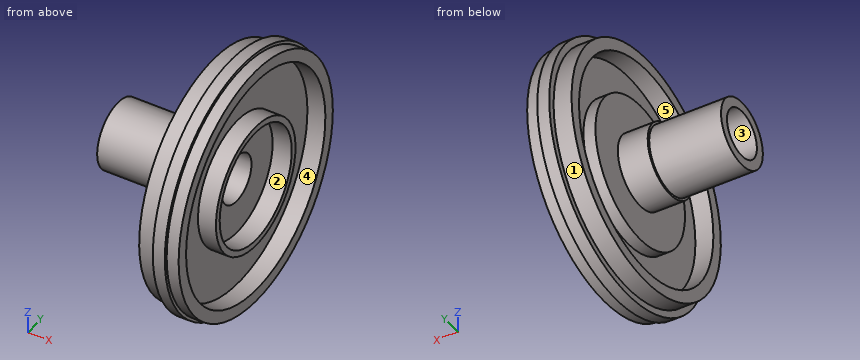
```python
from build123d import *


with BuildPart() as part:
    # Sketch1 → Revolve1 (revolve)
    with BuildSketch(Plane.XY, mode=Mode.PRIVATE) as revolve1_sk:
        Polygon((0, 6.35), (31.4198, 6.35), (31.4198, 15.33525), (36.4998, 15.33525), (36.4998, 16.92275), (31.7373, 16.92275), (31.7373, 29.62275), (36.4998, 29.62275), (36.4998, 32.79775), (33.3248, 32.79775), (33.3248, 33.5915), (30.1498, 33.5915), (30.1498, 31.75), (25.3873, 31.75), (25.3873, 28.575), (30.1498, 28.575), (30.1498, 19.05), (26.9748, 19.05), (26.9748, 9.525), (19.05, 9.525), (19.05, 8.89), (0, 8.89), align=None)
    revolve(revolve1_sk.sketch.rotate(Axis((0, 0, 0), (1, 0, 0)), 90), axis=Axis((0, 0, 0), (1, 0, 0)))


solid = part.part
```
Model file for the job. Use its own axes, mm. Face numbers are marked on the shaded views. A direction names the side the tool comes from. Coordinates: 2 decimals unless noted, no trailing zeros. Order: outer loops, then holes, each group sorted by start corner. A loop starts at its lowest first (then second) coordinate and runs counter-clockwise, first axis right, second up. Notation, with made-up numbers: (8.25, 32.25) - (12.25, 32.25) arc R20 cw to (12.25, 62.25) - close; hole circle Ø5 at (29, 24). An arc over 180 degrees is marked (long way). Return JSON: item names as keys, results as strings. Group by question number.
1) Saw through at D-D, the plane y = 18. Write the cut outline in (x, z).
2) Tool access for the marked faces 3, 4 and 5: list every direction of +Z, -Z, +X, -X, +Y, -Y with a clear straight run to the whole face (end or side of a thin tool).
3) Saw through at B-B, the plane x = 17.5. Write the cut outline in (y, z), plus the area to 3 significant figures.
4) Probe line 1 (Y direction, x = 33.8, z = 0); line 2 (Y direction, x = 33, z = 0); line 3 (Z direction, x = 26, y = -8.5). List the from-to ranges inside material, lowest first. Write a range as from..to.
5) Flat gauge pins, fed straight in: P1, Ø6, axis at y = 20, z = 15.5, coming from the -X side; P2, Ø1, axis at x = 24.5, y = 5.5, coming from the +Z side; P3, Ø6, axis at x = 4.5, y = 8, coming from the -Z side. Where does each tip first touch, or does it go through?
6) Saw through at C-C, the plane z = -26.5. Write the cut outline in (x, y).
7) Saw through at A-A, the plane x = 29. Write the cut outline in (y, z) (3 decimals), plus the area to 3 significant figures.
8) Mould opens along Z. For the marked faces 1 and 2 say: released by +Z, released by -Z, zero draft, split by the parting line, or undercut.
Values found:
{
 "1": {"outline": "(25.39, -26.15) - (30.15, -26.15) - (30.15, -28.36) - (33.32, -28.36) - (33.32, -27.42) - (36.5, -27.42) - (36.5, -23.53) - (31.74, -23.53) - (31.74, 23.53) - (36.5, 23.53) - (36.5, 27.42) - (33.32, 27.42) - (33.32, 28.36) - (30.15, 28.36) - (30.15, 26.15) - (25.39, 26.15) - (25.39, 22.19) - (30.15, 22.19) - (30.15, 6.24) - (26.97, 6.24) - (26.97, -6.24) - (30.15, -6.24) - (30.15, -22.19) - (25.39, -22.19) - close"},
 "2": {"face 3": "+X, -X", "face 4": "+X", "face 5": "-X"},
 "3": {"outline": "circle Ø17.78 at (0, 0); hole circle Ø12.7 at (0, 0)", "area": "122 mm²"},
 "4": {"line 1": "y = -32.8..-29.62, -16.92..-15.34, 15.34..16.92, 29.62..32.8", "line 2": "y = -33.59..-29.62, -16.92..-15.34, 15.34..16.92, 29.62..33.59", "line 3": "z = -30.59..-27.28, -4.3..4.3, 27.28..30.59"},
 "5": {"P1": "stops at x = 30.15", "P2": "stops at z = 8.11", "P3": "stops at z = -7.35"},
 "6": {"outline": "(25.39, -17.49) - (30.15, -17.49) - (30.15, -20.64) - (33.32, -20.64) - (33.32, -19.32) - (36.5, -19.32) - (36.5, -13.24) - (31.74, -13.24) - (31.74, 13.24) - (36.5, 13.24) - (36.5, 19.32) - (33.32, 19.32) - (33.32, 20.64) - (30.15, 20.64) - (30.15, 17.49) - (25.39, 17.49) - (25.39, 10.69) - (30.15, 10.69) - (30.15, -10.69) - (25.39, -10.69) - close"},
 "7": {"outline": "circle Ø63.5 at (0, 0); circle Ø38.1 at (0, 0); hole circle Ø57.15 at (0, 0); hole circle Ø12.7 at (0, 0)", "area": "1,620 mm²"},
 "8": {"face 1": "split by the parting line", "face 2": "undercut"}
}
